The drawing under review shows one solid part. Ordinate dimensions are in mm from its lowest x, y, z. Coordinates: 2 decimals unless noted, no trailing zeros. Write each loop counter-clockwise with the first axis right and the second up, starting at its lowest first coordinate (ties: lowest second). Pieces come first, ordered by that corner, then holes.
Q1. For probe 1 along Z at (x, y) = (2.25, 278.5); probe 2 along Y at (x, z) = (5.5, 79); probe 3 along Z at (x, y) = (11, 280) (1 decimal), list the stretches that pass through material, from the lowest coordinate up.
Q2. Take a section at C-C (z = 68.5). Give the boundary of the cut face in (x, y), and give its area (3 significant figures).
Q3. Take a section at B-B (z = 18). Give the boundary of the cut face in (x, y).
Q4. Insertion check: pin 1 (10 mm diameter, centred on x = 13, y = 268, fed in from +Z) (1 decimal). The pin has a flat end and moves straight along its axis. Give the tip position at first contact, or say it passes through.
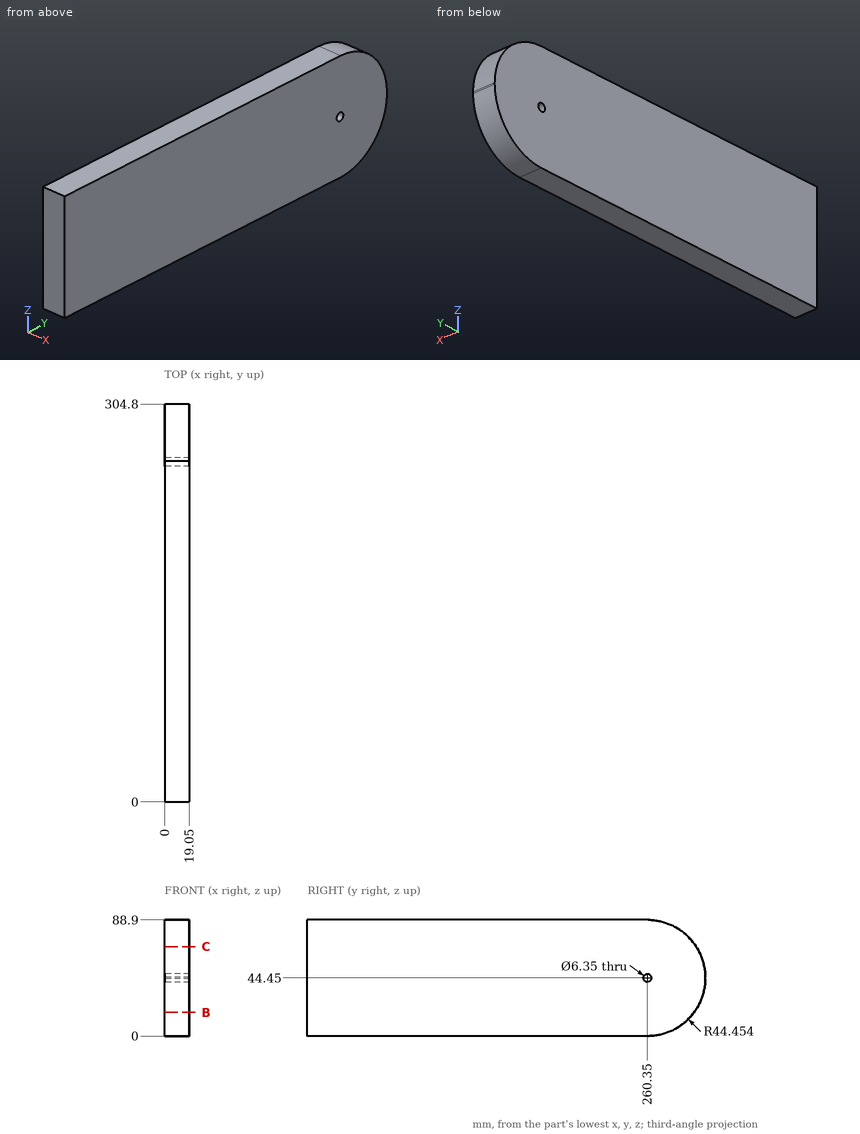
Response:
1. probe 1: z = 3.87 to 85.03
1. probe 2: y = 0 to 288.32
1. probe 3: z = 4.6 to 84.3
2. outline: (0, 0) - (19.05, 0) - (19.05, 297.74) - (0, 297.74) - close
2. area: 5,670 mm2
3. outline: (0, 0) - (19.05, 0) - (19.05, 296.08) - (0, 296.08) - close
4. pin 1: stops at z = 88.8
